For this review, take the finished solid that the model builds, in its own axes (mm). A direction names the side the tool comes from. Round coordinates to 2 decimals unless told otherwise and drop trailing zeros. Loops run counter-clockwise (first coordinate to the right, second up) from the corner with the lowest first, then second, coordinate; pieces in that order, holes last. Notation, with made-up numbers: M 20,38 L 30,38 A31 ccw 30,66 Z; hole C 83.25,-26.5 d6. An arc over 180 degrees is marked long. Write item = value, one per line. Start each with the question number.
```python
from build123d import *

# Parameters (mm, degrees)
SKETCH_1_W      = 49
SKETCH_1_H      = 26
EXTRUDE_1_DEPTH = 1.5
SKETCH_2_W      = 46
SKETCH_2_H      = 23
EXTRUDE_2_DEPTH = 1
FILLET_1_R      = 1


with BuildPart() as part:
    # 草图1 → 凸台-拉伸1 (new body)
    with BuildSketch(Plane(origin=(0, 0, 0), x_dir=(1, 0, 0), z_dir=(0, 1, 0))):
        Rectangle(SKETCH_1_W, SKETCH_1_H)
    extrude(amount=EXTRUDE_1_DEPTH)

    # 草图2 → 凸台-拉伸2 (add)
    with BuildSketch(Plane(origin=(0, 1.5, 0), x_dir=(1, 0, 0), z_dir=(0, 1, 0))):
        Rectangle(SKETCH_2_W, SKETCH_2_H)
    extrude(amount=EXTRUDE_2_DEPTH)

    # 圆角1
    fillet_1_edges = [part.edges().sort_by_distance(p)[0] for p in [
        (0, 0, 13),
        (-24.5, 0, 0),
        (0, 0, -13),
        (24.5, 0, 0),
    ]]
    fillet(fillet_1_edges, radius=FILLET_1_R)


solid = part.part
```
(1) Wall thickness on L1, parallel to X at y = 1.65, z = -7.5; L2, parallel to Z at x = -21.5, y = 2.2; L3, parallel to X at y = 0.95, z = 7.5: over which ranges is each line inside the solid? List them lowest first.
(2) Tool access review of faces 1 (the flat face through (0, 2, -11.5)), 2 (the flat face through (23, 2, 0)), 3 (the flat face through (0, 2, 11.5)): name each direction out of +Z, -Z, +X, -X, +Y, -Y from which nothing blocks a thin tool from reaching the whole face with its end or side.
(3) Add section B-B on x = -8. Write out the cut boundary in (y, z).
(4) Add section A-A on z = 2.75. Write out the cut boundary in (x, y).
(5) Add section C-C on y = 2. Write out the cut boundary in (x, z), and give its area (3 significant figures).
(6) For pin 1 Ø0.8 at (x, y) = (-2, 2) entering from -Z; pin 2 Ø0.5 at (x, y) = (11, 2) entering from +Z; pin 3 Ø1.1 at (y, z) = (2, 2.5) entering from +X, all flat-tipped, find the tip position at first contact; note any pin that passes through.
Answer sheet:
q1.L1 = -23 to 23
q1.L2 = -11.5 to 11.5
q1.L3 = -24.5 to 24.5
q2.face_1 = -Z, +X, -X, +Y
q2.face_2 = +Z, -Z, +X, +Y
q2.face_3 = +Z, +X, -X, +Y
q3.outline = M 0,-12 A1 ccw 1,-13 L 1.5,-13 L 1.5,-11.5 L 2.5,-11.5 L 2.5,11.5 L 1.5,11.5 L 1.5,13 L 1,13 A1 ccw 0,12 Z
q4.outline = M -24.5,1 A1 ccw -23.5,0 L 23.5,0 A1 ccw 24.5,1 L 24.5,1.5 L 23,1.5 L 23,2.5 L -23,2.5 L -23,1.5 L -24.5,1.5 Z
q5.outline = M -23,-11.5 L 23,-11.5 L 23,11.5 L -23,11.5 Z
q5.area = 1,060 mm²
q6.pin_1 = -11.5
q6.pin_2 = 11.5
q6.pin_3 = 24.5
